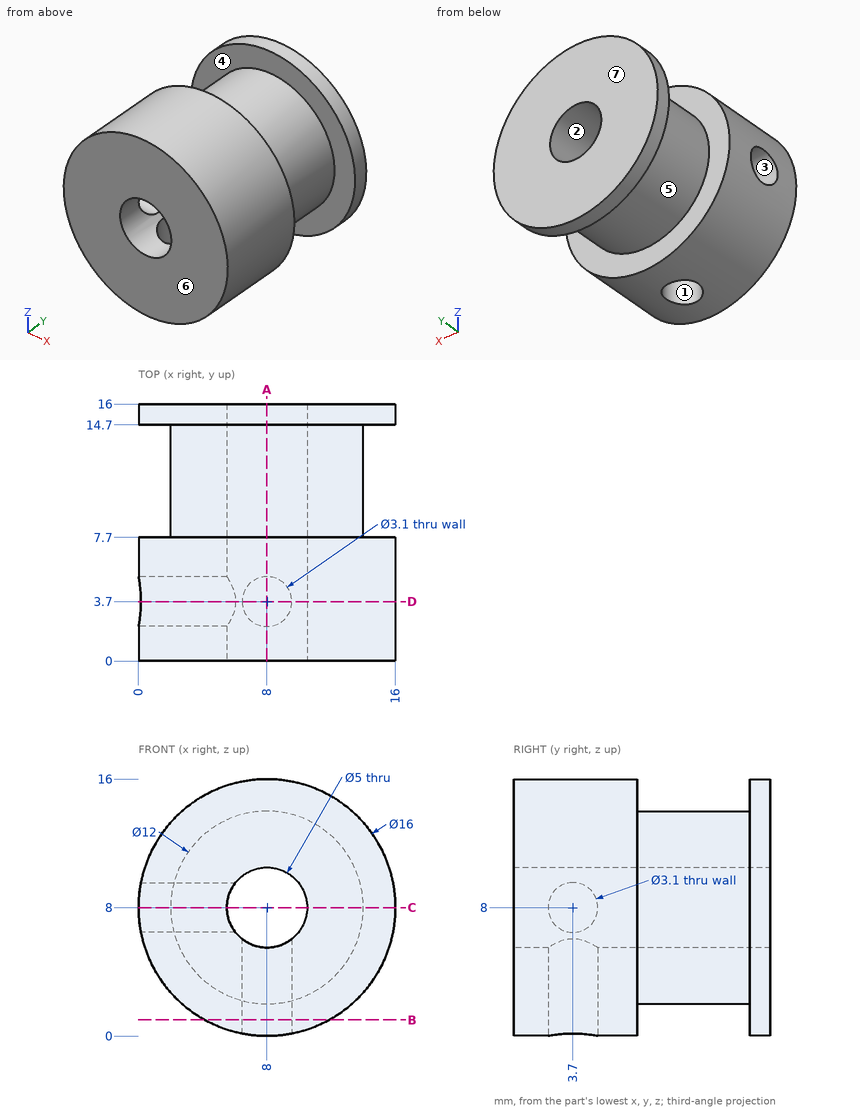
Drawing for the job (mm, zero at the part's lowest x, y, z). A direction names the side the tool comes from. Give positions to 0.01 mm unless a question says otherwise; leave off trailing zeros. Write each loop counter-clockwise with the first axis right and the second up, starting at its lowest first coordinate (ties: lowest second). Pieces come first, ordered by that corner, then holes. Notation, with made-up numbers: M -21,11.25 L 12,11.25 A22 ccw 12,22.25 Z; hole C 13,-1.75 d6. An arc over 180 degrees is marked long. Use CSV: the item, a comma, the result in double quotes.
Item 1: Which spindle directions (+Z, -Z, +X, -X, +Y, -Y) get a long thin tool onto all of the face, cutting with end or side? Do the marked faces 1, 2, 3 and 4. Say none if no direction does.
Taken from the geometry:
face 1,"-Z"
face 2,"+Y, -Y"
face 3,"-X"
face 4,"none"
Item 2: Pull direction Y, two halves, no side cores. Call the marked faces 5, 6 and 7: +Y half, -Y half, draft (parallel to the pull), parting line (faces both ways), or undercut.
Taken from the geometry:
face 5,"undercut"
face 6,"-Y half"
face 7,"+Y half"
Item 3: Slice it at C-C on z = 8. Write the cut outline in (x, y).
Taken from the geometry:
outline,"M 0,0 L 5.5,0 L 5.5,2.15 L 0,2.15 Z; M 0,5.25 L 5.5,5.25 L 5.5,16 L 0,16 L 0,14.7 L 2,14.7 L 2,7.7 L 0,7.7 Z; M 10.5,0 L 16,0 L 16,7.7 L 14,7.7 L 14,14.7 L 16,14.7 L 16,16 L 10.5,16 Z"
Item 4: Pin check, flat tips, straight feed: P1, Ø1, axis at y = 7, z = 13, coming from the +X side; P2, Ø1, axis at y = 11.5, z = 3.5, coming from the -X side; P3, Ø6, axis at y = 7.5, z = 2.5, coming from the -X side. Stop position of each tip, or through.
Taken from the geometry:
P1,"stops at x = 14.61"
P2,"stops at x = 3.53"
P3,"stops at x = 0.4"
Item 5: Slice it at A-A on x = 8. Write the cut outline in (y, z), plus the area to 3 significant figures.
Taken from the geometry:
outline,"M 0,0 L 2.15,0 L 2.15,5.5 L 0,5.5 Z; M 0,10.5 L 16,10.5 L 16,16 L 14.7,16 L 14.7,14 L 7.7,14 L 7.7,16 L 0,16 Z; M 5.25,0 L 7.7,0 L 7.7,2 L 14.7,2 L 14.7,0 L 16,0 L 16,5.5 L 5.25,5.5 Z"
area,"131 mm²"
Item 6: Drill centre lines: probe 1 along X at (y, z) = (8.25, 8); probe 2 along Y at (x, z) = (4.25, 8); probe 3 along Y at (x, z) = (5.75, 15.5). Where is each one in solid material? Low to high.
Taken from the geometry:
probe 1,"x = 2 to 5.5, 10.5 to 14"
probe 2,"y = 0 to 2.15, 5.25 to 16"
probe 3,"y = 0 to 7.7, 14.7 to 16"
Item 7: Slice it at B-B on z = 1. Write the cut outline in (x, y), plus the area to 3 significant figures.
Taken from the geometry:
outline,"M 4.13,0 L 11.87,0 L 11.87,7.7 L 4.13,7.7 Z; M 4.13,14.7 L 11.87,14.7 L 11.87,16 L 4.13,16 Z; hole C 8,3.7 d3.1"
area,"62.2 mm²"
Item 8: Slice it at D-D on y = 3.7. Write the cut outline in (x, z), plus the area to 3 significant figures.
Taken from the geometry:
outline,"M 0.15,6.45 A8 ccw 6.45,0.15 L 6.45,6.04 A2.5 cw 6.04,6.45 Z; M 0.15,9.55 L 6.04,9.55 A2.5 cw long 9.55,6.04 L 9.55,0.15 A8 ccw long Z"
area,"147 mm²"
